Here's the drawing with two shaded views (mm, measured from the low corner). I have some questions. A direction names the side the tool comes from. Give positions to 0.01 mm unless a question says otherwise; leave off trailing zeros. Loops run counter-clockwise (first coordinate to the right, second up) from the corner with the lowest first, then second, coordinate; pieces in that order, holes last. Notation, with made-up numbers: M 28,34 L 45,34 A30 ccw 45,56 Z; hole C 76.5,84 d4. An arc over 180 degrees is marked long. Use a Markdown table: item, result. Add a question column.
1) If I drill on line 1 along X through (y, z) = (0.2, 4.3); line 2 along Y through (x, z) = (6, 4.35), over which ranges is the centre line in solid material (lowest first)? Write a range as [from, to].
2) Suppose I cut it at A-A on y = 1.15. List the corners of the cut face in (x, z) for me.
3) We'd pull the mould along Z, two halves only. Please class the marked faces 4, 5, 6 and 7: +Z half, -Z half, draft (parallel to the pull), parting line (faces both ways), or undercut.
4) Suppose I cut it at C-C on z = 0.8. List the corners of the cut face in (x, y) for me, and give its area (3 significant figures).
5) Suppose I cut it at D-D on x = 5.75. List the corners of the cut face in (y, z) for me.
6) Will these pins go through, and if not, where does the flat tip stop? pin 1 Ø1.5 at (x, z) = (1.5, 2.5) entering from -Y; pin 2 Ø1 at (x, y) = (2.5, 1) entering from -Z.
7) Suppose I cut it at B-B on x = 9.5. List the corners of the cut face in (y, z) for me, and give its area (3 significant figures).
8) Which directions (+Z, -Z, +X, -X, +Y, -Y) give clear straight access to the entire face, cutting with the end or side of a thin tool? Please do the marked faces 1, 2 and 3.
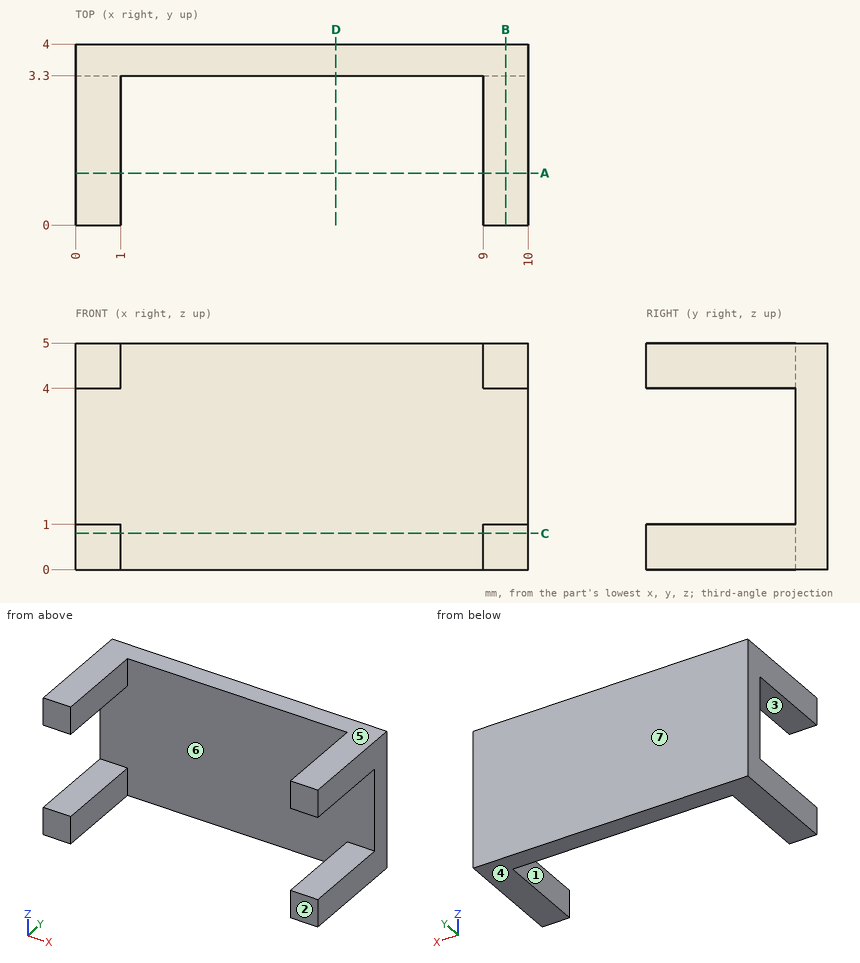
Answer block:
| question | item | result |
|---|---|---|
| 1 | line 1 | x = [0, 1], [9, 10] |
| 1 | line 2 | y = [3.3, 4] |
| 2 | outline | M 0,0 L 1,0 L 1,1 L 0,1 Z; M 0,4 L 1,4 L 1,5 L 0,5 Z; M 9,0 L 10,0 L 10,1 L 9,1 Z; M 9,4 L 10,4 L 10,5 L 9,5 Z |
| 3 | face 4 | -Z half |
| 3 | face 5 | +Z half |
| 3 | face 6 | undercut |
| 3 | face 7 | draft |
| 4 | outline | M 0,0 L 1,0 L 1,3.3 L 9,3.3 L 9,0 L 10,0 L 10,4 L 0,4 Z |
| 4 | area | 13.6 mm^2 |
| 5 | outline | M 3.3,0 L 4,0 L 4,5 L 3.3,5 Z |
| 6 | pin 1 | stops at y = 3.3 |
| 6 | pin 2 | passes through |
| 7 | outline | M 0,0 L 4,0 L 4,5 L 0,5 L 0,4 L 3.3,4 L 3.3,1 L 0,1 Z |
| 7 | area | 10.1 mm^2 |
| 8 | face 1 | +Z, -Z, -Y |
| 8 | face 2 | +Z, -Z, +X, -X, -Y |
| 8 | face 3 | +X, -X, -Y |
